Build history of the part. All positions in model axes, mm. A direction names the side the tool comes from. Round coordinates to 2 decimals unless told otherwise and drop trailing zeros. Order: outer loops, then holes, each group sorted by start corner. A loop starts at its lowest first (then second) coordinate and runs counter-clockwise, first axis right, second up. Notation, with made-up numbers: (-12, 25.25) - (19, 25.25) arc R27 ccw to (19, 59.25) - close; hole circle Ø1 at (6, -27). An arc over 180 degrees is marked (long way). Write each question's results on one line, items separated by ' | '. Start each with the question number.
```python
from build123d import *

# Parameters (mm, degrees)
BOSS_EXTRUDE1_DEPTH    = 38.1
CONVERT_SOLID1_DEPTH   = 38.1
CONVERT_SOLID1_2_DEPTH = 38.1


# Read off the part's stored shape, not the designer's step: Convert-Solid1
with BuildPart() as part:
    # Sketch1 → Boss-Extrude1 (new body)
    with BuildSketch(Plane.XY):
        Polygon((-38.191130673, 27.446595767), (-38.191130673, 0), (-11.295536696, 0), (-11.295536696, 26.723586817), (-9.263536696, 26.723586817), (-9.263536696, -2.032), (-40.223130673, -2.032), (-40.223130673, 27.446595767), align=None)
    extrude(amount=BOSS_EXTRUDE1_DEPTH)

    # Convert-Solid1 outline → Convert-Solid1 (cut)
    with BuildSketch(Plane.XY):
        with BuildLine():
            Line((-9.263536696, -2.032), (-9.263536696, 2.728000132))
            ThreePointArc((-9.263536696, 2.728000132), (-10.657708456, -0.63782824), (-14.023536828, -2.032))
            Line((-14.023536828, -2.032), (-9.263536696, -2.032))
        make_face()
        with BuildLine():
            Line((-40.223130673, -2.032), (-35.463130541, -2.032))
            ThreePointArc((-35.463130541, -2.032), (-38.828958913, -0.63782824), (-40.223130673, 2.728000132))
            Line((-40.223130673, 2.728000132), (-40.223130673, -2.032))
        make_face()
    extrude(amount=CONVERT_SOLID1_DEPTH, mode=Mode.SUBTRACT)

    # Convert-Solid1 2 outline → Convert-Solid1 2 (add)
    with BuildSketch(Plane.XY):
        with BuildLine():
            Line((-11.295536696, 0), (-11.295536696, 26.723586817))
            Line((-11.295536696, 26.723586817), (-11.643536762, 26.723586817))
            Line((-11.643536762, 26.723586817), (-11.643536762, 2.728000132))
            ThreePointArc((-11.643536762, 2.728000132), (-12.340622642, 1.045085946), (-14.023536828, 0.348000066))
            Line((-14.023536828, 0.348000066), (-35.463130541, 0.348000066))
            ThreePointArc((-35.463130541, 0.348000066), (-37.146044727, 1.045085946), (-37.843130607, 2.728000132))
            Line((-37.843130607, 2.728000132), (-37.843130607, 27.446595767))
            Line((-37.843130607, 27.446595767), (-38.191130673, 27.446595767))
            Line((-38.191130673, 27.446595767), (-38.191130673, 0))
            Line((-38.191130673, 0), (-11.295536696, 0))
        make_face()
    extrude(amount=CONVERT_SOLID1_2_DEPTH)


solid = part.part
```
1. Mould opens along X. For faces 3 (the face through (-10, 26.724, 19)), 4 (the face through (-10.62, -0.6, 18.78)), 5 (the face through (-11.644, 15, 19)) say: pulls with the +X half, pulls with the -X half, needs draft (parallel to the pull), parting line crosses it, or undercut.
2. Cut at B-B (z = 27). List the corners of the cut face in (x, y), plus the area to 3 significant figures.
3. 3-axis set-ups, long thin cutter, end or side, ignore diameter. For faces 1 (the face through (-25, 0, 38.1)), 2 (the face through (-37.843, 15, 19)): which of +Z, -Z, +X, -X, +Y, -Y reach the whole face in a straight line?
4. Cut at C-C (x = -24). List the corners of the cut face in (y, z).
5. Wall check: line 1 (X direction, y = 3.5, z = 10); line 2 (Y direction, x = -22, z = 32.5); line 3 (Y direction, x = -12, z = 27). Give the ranges that are in metal, low to high. Write a range as from..to.
6. Cut at A-A (y = 24). List the corners of the cut face in (x, z).
7. Cut at D-D (x = -13). List the corners of the cut face in (y, z).
8. Flat gauge pins, fed straight in: pin 1 Ø3 at (x, z) = (-23.5, 24.5) entering from +Y; pin 2 Ø17 at (x, z) = (-27.5, 22) entering from +Y; pin 3 Ø1.2 at (x, z) = (-10, 10.5) entering from +Y; pin 4 Ø10 at (x, y) = (-15, 22.5) entering from -Z. Where does each tip first touch, or does it go through?
A:
1) face 3: needs draft | face 4: pulls with the +X half | face 5: undercut
2) outline: (-40.22, 2.73) arc R4.76 ccw to (-35.46, -2.03) - (-14.02, -2.03) arc R4.76 ccw to (-9.26, 2.73) - (-9.26, 26.72) - (-11.64, 26.72) - (-11.64, 2.73) arc R2.38 cw to (-14.02, 0.35) - (-35.46, 0.35) arc R2.38 cw to (-37.84, 2.73) - (-37.84, 27.45) - (-40.22, 27.45) - close | area: 194 mm^2
3) face 1: +Z, +X, -X, +Y, -Y | face 2: +Z, -Z, +Y
4) outline: (-2.03, 0) - (0.35, 0) - (0.35, 38.1) - (-2.03, 38.1) - close
5) line 1: x = -40.22..-37.84, -11.64..-9.26 | line 2: y = -2.03..0.35 | line 3: y = -1.58..1.48
6) outline: (-40.22, 0) - (-37.84, 0) - (-37.84, 38.1) - (-40.22, 38.1) - close; (-11.64, 0) - (-9.26, 0) - (-9.26, 38.1) - (-11.64, 38.1) - close
7) outline: (-1.92, 0) - (0.58, 0) - (0.58, 38.1) - (-1.92, 38.1) - close
8) pin 1: stops at y = 0.35 | pin 2: stops at y = 0.41 | pin 3: stops at y = 26.72 | pin 4: stops at z = 0
